For this review, take the finished solid that the model builds, in its own axes (mm). A direction names the side the tool comes from. Round coordinates to 2 decimals unless told otherwise and drop trailing zeros. Order: outer loops, then holes, each group sorted by start corner. A loop starts at its lowest first (then second) coordinate and runs counter-clockwise, first axis right, second up. Notation, with made-up numbers: M -13.5,-7.5 L -1.5,-7.5 A6 cw -1.5,-1.5 Z; hole C -36,40 d4. An arc over 180 degrees is marked long. Put each result on its own line as item: value.
from build123d import *

# Parameters (mm, degrees)
BOX001_W            = 3
BOX001_H            = 1
BOX001_DEPTH        = 5
CYLINDER_R          = 3.5
CYLINDER_DEPTH      = 2
CYLINDER_ROLL_ANGLE = 90
BOX_W               = 10
BOX_H               = 20
BOX_DEPTH           = 10


with BuildPart() as cube:
    # Box001 → Box001 (new body)
    with BuildSketch(Plane(origin=(3.5, 0, 5), x_dir=(1, 0, 0), z_dir=(0, 0, 1))):
        with Locations((1.5, 0.5)):
            Rectangle(BOX001_W, BOX001_H)
    extrude(amount=BOX001_DEPTH)


with BuildPart() as solenoid_head_slot:
    # Cylinder → Cylinder (new body)
    with BuildSketch(Plane.XY):
        Circle(CYLINDER_R)
    extrude(amount=CYLINDER_DEPTH)


with BuildPart() as solenoid_head_slot_1:
    # Cylinder roll: moved
    add(solenoid_head_slot.part.rotate(Axis((0, 0, 0), (1, 0, 0)), CYLINDER_ROLL_ANGLE))


with BuildPart() as solenoid_head_slot_2:
    # Cylinder placement: moved
    add(solenoid_head_slot_1.part.moved(Location((5, 3, 8))))


with BuildPart() as cut001:
    # Box → Box (new body)
    with BuildSketch(Plane.XY):
        with Locations((5, 10)):
            Rectangle(BOX_W, BOX_H)
    extrude(amount=BOX_DEPTH)

    # Cut: cut solenoid_head_slot
    add(solenoid_head_slot_2.part, mode=Mode.SUBTRACT)

    # Cut001: cut Cube
    add(cube.part, mode=Mode.SUBTRACT)


solid = cut001.part
(1) Draft analysis for pull direction Y (two halves, no side actions). For faces 1 (the face through (5, 10, 0)), 2 (the face through (5, 0, 4)), 3 (the face through (5, 3, 7)), state which applies: released by +Y, released by -Y, zero draft, split by the parting line, or undercut.
A:
face 1: zero draft
face 2: released by -Y
face 3: undercut
(2) For faces 4 (the face through (4.9, 2, 4.5)), 5 (the face through (0, 10, 5)), 6 (the face through (3.5, 0.5, 7.5)), list the 3-axis set-ups (+Z, -Z, +X, -X, +Y, -Y) from which the entire face can be reached by the end or side of a thin tool; tool diameter is ignored.
A:
face 4: none
face 5: +Z, -Z, -X, +Y, -Y
face 6: +Z, -Y
(3) Add section A-A on x = 5. Give the boundary of the cut face in (y, z), then the cut area to 3 significant figures.
A:
outline: M 0,0 L 20,0 L 20,10 L 3,10 L 3,4.5 L 1,4.5 L 1,5 L 0,5 Z
area: 184 mm2
(4) To check wall thickness, follow L1, parallel to Y at x = 2.75, z = 5.75; L2, parallel to X at y = 2.65, z = 8; L3, parallel to Y at x = 5, z = 8.75. State the ranges of each line that lie inside material, in increasing order.
A:
L1: y = 0 to 1, 3 to 20
L2: x = 0 to 1.5, 8.5 to 10
L3: y = 3 to 20
(5) Add section B-B on z = 8. Give the boundary of the cut face in (x, y), then the cut area to 3 significant figures.
A:
outline: M 0,0 L 3.5,0 L 3.5,1 L 1.5,1 L 1.5,3 L 8.5,3 L 8.5,1 L 6.5,1 L 6.5,0 L 10,0 L 10,20 L 0,20 Z
area: 183 mm2
(6) Add section C-C on x = 1.75. Give the boundary of the cut face in (y, z), then the cut area to 3 significant figures.
A:
outline: M 0,0 L 20,0 L 20,10 L 0,10 Z; hole M 1,6.7 L 3,6.7 L 3,9.3 L 1,9.3 Z
area: 195 mm2
(7) Insertion check: pin 1 Ø1.1 at (x, y) = (4.5, 0.5) entering from +Z. The pin has a flat end and moves straight along its axis. Give the tip position at first contact, or say it passes through.
A:
pin 1: stops at z = 5
(8) Add section D-D on z = 7. Give the boundary of the cut face in (x, y), then the cut area to 3 significant figures.
A:
outline: M 0,0 L 3.5,0 L 3.5,1 L 1.65,1 L 1.65,3 L 8.35,3 L 8.35,1 L 6.5,1 L 6.5,0 L 10,0 L 10,20 L 0,20 Z
area: 184 mm2
